Source: three-view drawing plus pictorial views. Frame: mm from the lowest corner of the part. A direction names the side the tool comes from. Give positions to 0.01 mm unless a question says otherwise; leave off trailing zeros. Order: outer loops, then holes, each group sorted by start corner. A loop starts at its lowest first (then second) coordinate and runs counter-clockwise, first axis right, second up.
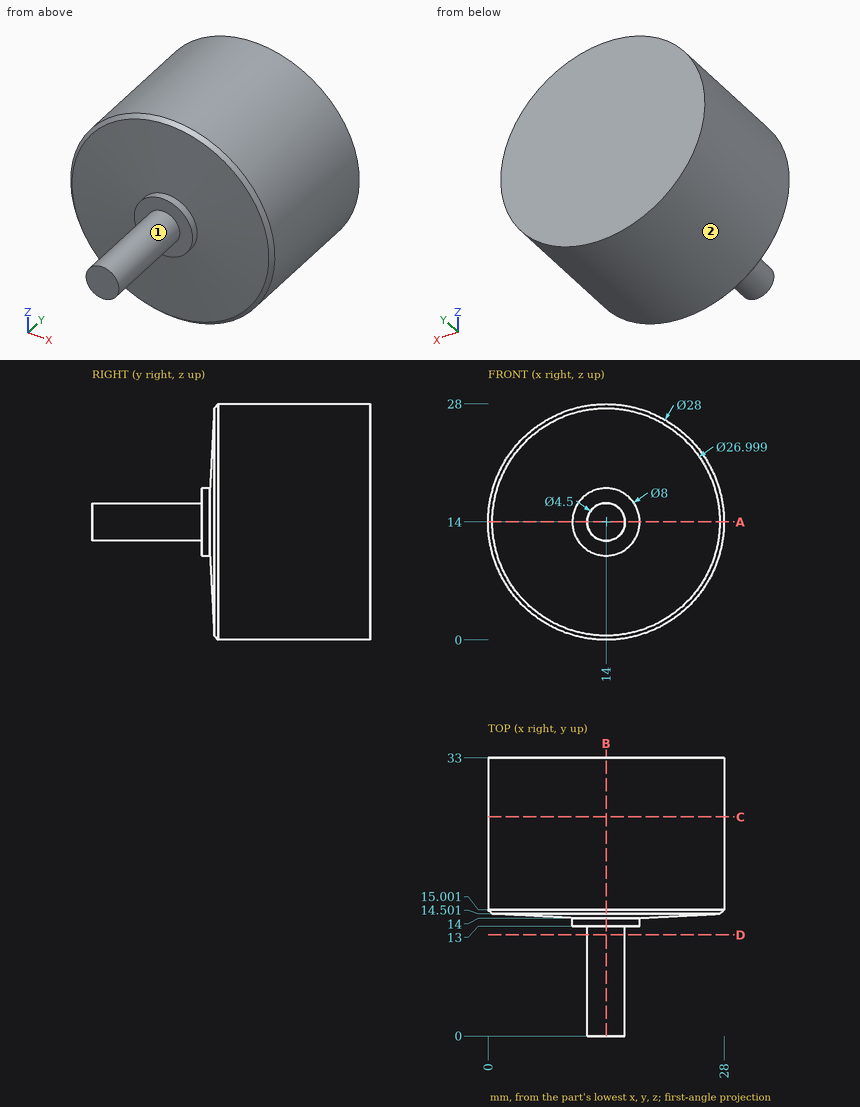
1) Reachability of the marked faces 1 and 2 from +Z, -Z, +X, -X, +Y, -Y: full face, straight path, thin tool, end or side. Return the list, or none.
Checks:
face 1: -Y
face 2: +Y, -Y
2) Section query D-D on y = 12. Output: boundary loops of the cut face in (x, z), and give its area (3 significant figures).
Checks:
outline: circle Ø4.5 at (14, 14)
area: 15.9 mm2
3) First-contact query: pin 1 Ø3 at (y, z) = (27.5, 7.5) entering from +X; pin 2 Ø8 at (y, z) = (4.5, 21) entering from +X; pin 3 Ø12 at (x, y) = (23, 9) entering from -Z (1 decimal). Flat tips, straight axial feed; report the tip coordinate or a pass-through.
Checks:
pin 1: stops at x = 27.08
pin 2: passes through
pin 3: stops at z = 2.2
4) Section query C-C on y = 26. Output: boundary loops of the cut face in (x, z).
Checks:
outline: circle Ø28 at (14, 14)
5) Section query B-B on x = 14. Output: boundary loops of the cut face in (y, z).
Checks:
outline: (0, 11.75) - (13, 11.75) - (13, 10) - (14, 10) - (14.5, 0.5) - (15, 0) - (33, 0) - (33, 28) - (15, 28) - (14.5, 27.5) - (14, 18) - (13, 18) - (13, 16.25) - (0, 16.25) - close
6) Ray query, L1, parallel to X at y = 26, z = 11.5 (1 decimal); L2, parallel to X at y = 28, z = 26.75 (1 decimal); L3, parallel to Y at x = 19.25, z = 14.5. Return the intervals inside material, ascending.
Checks:
L1: x = 0.2 to 27.8
L2: x = 8.2 to 19.8
L3: y = 14.07 to 33
7) Section query A-A on z = 14. Output: boundary loops of the cut face in (x, y).
Checks:
outline: (0, 15) - (0.5, 14.5) - (10, 14) - (10, 13) - (11.75, 13) - (11.75, 0) - (16.25, 0) - (16.25, 13) - (18, 13) - (18, 14) - (27.5, 14.5) - (28, 15) - (28, 33) - (0, 33) - close
